from build123d import *

# Parameters (mm, degrees)
F0_W     = 152.4
F0_H     = 25.4
F1_DEPTH = 3.175
F2_W     = 25.4
F2_H     = 3.175
F3_DEPTH = 152.4
F4_W     = 76.2
F4_H     = 22.225
F5_DEPTH = 3.175


# Not quite as in the source:
# - a length typed as a fraction of an inch, garbled in the dataset ("3 / 203.2 mm" for 3/8 in), is restored


with BuildPart() as f1:
    # F0 (on Front) → F1 (new body)
    with BuildSketch(Plane.XZ):
        with Locations((48.1263138257, 41.5133684874)):
            Rectangle(F0_W, F0_H)
    extrude(amount=F1_DEPTH)

    # F2 (on face) → F3 (join)
    with BuildSketch(Plane.YZ.offset(124.3263138257)):
        with Locations((-15.875, 30.4008684874)):
            Rectangle(F2_W, F2_H)
    extrude(amount=-F3_DEPTH)

    # F4 (on face) → F5 (join)
    with BuildSketch(Plane.XZ.offset(28.575)):
        with Locations((10.0263138257, 17.7008684874)):
            Rectangle(F4_W, F4_H)
    extrude(amount=-F5_DEPTH)


solid = f1.part
For this review, take the finished solid that the model builds, in its own axes (mm). A direction names the side the tool comes from. Round coordinates to 2 decimals unless told otherwise and drop trailing zeros. Write each loop counter-clockwise with the first axis right and the second up, starting at its lowest first coordinate (ties: lowest second). Pieces come first, ordered by that corner, then holes. Notation, with made-up numbers: (58, 71.25) - (89, 71.25) arc R23 cw to (89, 85.25) - close; hole circle Ø4 at (78, 67). An arc over 180 degrees is marked (long way). Write item = value, one per line. Start each with the question number.
1. Consider section C-C on y = -22.25. State the section outline as (x, z) points, plus the area to 3 significant figures.
2. Wall thickness on L1, parallel to Z at x = 114, y = -15; L2, parallel to Y at x = -19.5, z = 34.5 (3 decimals); L3, parallel to Z at x = 96.5, y = -1: over which ranges is each line inside the solid? List them lowest first.
3. For pin 1 Ø3.5 at (y, z) = (-27, 21) entering from +X; pin 2 Ø12 at (x, y) = (6.5, -17) entering from -Z; pin 3 Ø5 at (x, y) = (28.5, -23) entering from +Z, all flat-tipped, find the tip position at first contact; note any pin that passes through.
4. Consider section A-A on x = 81. State the section outline as (y, z) points (3 decimals).
5. Consider section B-B on z = 16. State the section outline as (x, y) points (3 decimals).
6. For faces 1 (the face through (124.326, -8, 31)), 2 (the face through (9, -25.4, 18)), 3 (the face through (47, -2, 54.213)), 4 (the face through (47, -3.175, 43)), 5 (the face through (48.126, -27, 18)), list the 3-axis set-ups (+Z, -Z, +X, -X, +Y, -Y) from which the entire face can be reached by the end or side of a thin tool; tool diameter is ignored.
7. Draft analysis for pull direction Z (two halves, no side actions). For faces 6 (the face through (13, -28.575, 19)), 7 (the face through (9, -27, 6.588)), 8 (the face through (49, -16, 31.988)), state which applies: released by +Z, released by -Z, zero draft, split by the parting line, or undercut.
8. Consider section D-D on x = 34. State the section outline as (y, z) points (3 decimals), plus the area to 3 significant figures.
Evaluation:
q1.outline = (-28.07, 28.81) - (124.33, 28.81) - (124.33, 31.99) - (-28.07, 31.99) - close
q1.area = 484 mm2
q2.L1 = 28.81 to 31.99
q2.L2 = -3.175 to 0
q2.L3 = 28.81 to 54.21
q3.pin_1 = 48.13
q3.pin_2 = 28.81
q3.pin_3 = 31.99
q4.outline = (-28.575, 28.813) - (0, 28.813) - (0, 54.213) - (-3.175, 54.213) - (-3.175, 31.988) - (-28.575, 31.988) - close
q5.outline = (-28.074, -28.575) - (48.126, -28.575) - (48.126, -25.4) - (-28.074, -25.4) - close
q6.face_1 = +Z, -Z, +X, +Y, -Y
q6.face_2 = -Z, +X, -X, +Y
q6.face_3 = +Z, +X, -X, +Y, -Y
q6.face_4 = +Z, +X, -X, -Y
q6.face_5 = -Z, +X, +Y, -Y
q7.face_6 = zero draft
q7.face_7 = released by -Z
q7.face_8 = released by +Z
q8.outline = (-28.575, 6.588) - (-25.4, 6.588) - (-25.4, 28.813) - (0, 28.813) - (0, 54.213) - (-3.175, 54.213) - (-3.175, 31.988) - (-28.575, 31.988) - close
q8.area = 232 mm2
